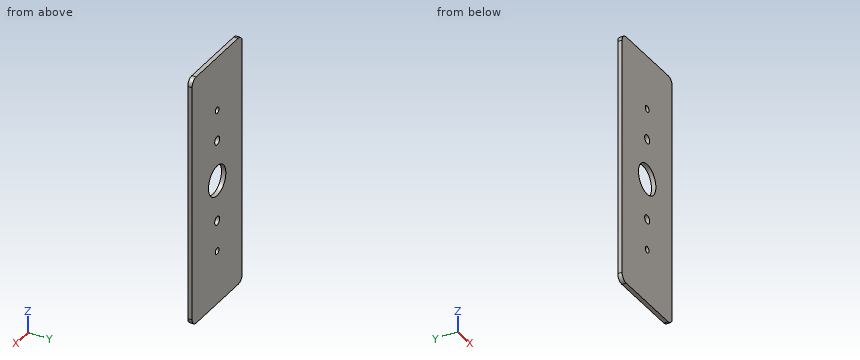
from build123d import *

# Parameters (mm, degrees)
SKETCH1_W               = 30.95625
SKETCH1_H               = 88.9
BOSS_EXTRUDE1_DEPTH     = 1.524
FILLET1_R               = 2.54
SKETCH6_R               = 1.524
CUT_EXTRUDE1_DEPTH      = 2.524
F_4_40_TAPPED_HOLE1_D   = 2.2606
F_1_2_13_TAPPED_HOLE1_D = 10.71626


with BuildPart() as part:
    # Sketch1 → Boss-Extrude1 (new body)
    with BuildSketch(Plane(origin=(0, 0, 0), x_dir=(1, 0, 0), z_dir=(0, 1, 0))):
        Rectangle(SKETCH1_W, SKETCH1_H)
    extrude(amount=BOSS_EXTRUDE1_DEPTH)

    # Fillet1
    fillet1_edges = [part.edges().sort_by_distance(p)[0] for p in [
        (15.478125, 0.762, -44.45),
        (15.478125, 0.762, 44.45),
        (-15.478125, 0.762, 44.45),
        (-15.478125, 0.762, -44.45),
    ]]
    fillet(fillet1_edges, radius=FILLET1_R)

    # Sketch6 → Cut-Extrude1 (cut, through all)
    with BuildSketch(Plane.XZ):
        with Locations((0, 14.478)):
            Circle(SKETCH6_R)
        with Locations((0, -14.478)):
            Circle(SKETCH6_R)
    extrude(amount=-CUT_EXTRUDE1_DEPTH, mode=Mode.SUBTRACT)

    # #4-40 Tapped Hole1 (through all)
    with Locations(Plane(origin=(0, 1.524, 0), x_dir=(-1, 0, 0), z_dir=(0, 1, 0))):
        with Locations((0, 25.4), (0, -25.4)):
            Hole(F_4_40_TAPPED_HOLE1_D / 2)

    # 1/2-13 Tapped Hole1 (through all)
    with Locations(Plane(origin=(0, 1.524, 0), x_dir=(-1, 0, 0), z_dir=(0, 1, 0))):
        with Locations((0, 0)):
            Hole(F_1_2_13_TAPPED_HOLE1_D / 2)


solid = part.part
Can you work these out from the model? Positions are in its coordinate system, mm. Coordinates: 2 decimals unless noted, no trailing zeros. Order: outer loops, then holes, each group sorted by start corner. A loop starts at its lowest first (then second) coordinate and runs counter-clockwise, first axis right, second up. Notation, with made-up numbers: (-25, -14) - (13, -14) arc R3 ccw to (13, -9) - close; hole circle Ø4 at (76, -15.75). An arc over 180 degrees is marked (long way). Answer as a JSON object with one key per item and string values. Group by question number.
Q1. Imagine slicing it at A-A (x = 0). Please give me the cut outline in (y, z), and give its area (3 significant figures).
Q2. Will this pin go through, and if not, where does the flat tip stop? P1, Ø1.8, axis at x = 0, z = 14.478, coming from the -Y side.
Q3. Imagine slicing it at B-B (z = 0). Please give me the cut outline in (x, y), and give its area (3 significant figures).
Q4. Imagine slicing it at C-C (x = -3.5). Please give me the cut outline in (y, z).
Q5. Imagine slicing it at D-D (y = 1.15). Please give me the cut outline in (x, z).
Q6. I need wall thicknesses on line 1 (Z direction, x = 0, y = 0.3); line 2 (Z direction, x = 3, y = 0.85). Which ranges of each line are inside material? Lowest first, please. Write a range as from..to.
Determined:
{
 "1": {"outline": "(0, -44.45) - (1.52, -44.45) - (1.52, -26.53) - (0, -26.53) - close; (0, -24.27) - (1.52, -24.27) - (1.52, -16) - (0, -16) - close; (0, -12.95) - (1.52, -12.95) - (1.52, -5.36) - (0, -5.36) - close; (0, 5.36) - (1.52, 5.36) - (1.52, 12.95) - (0, 12.95) - close; (0, 16) - (1.52, 16) - (1.52, 24.27) - (0, 24.27) - close; (0, 26.53) - (1.52, 26.53) - (1.52, 44.45) - (0, 44.45) - close", "area": "103 mm2"},
 "2": {"P1": "passes through"},
 "3": {"outline": "(-15.48, 0) - (-5.36, 0) - (-5.36, 1.52) - (-15.48, 1.52) - close; (5.36, 0) - (15.48, 0) - (15.48, 1.52) - (5.36, 1.52) - close", "area": "30.8 mm2"},
 "4": {"outline": "(0, -44.45) - (1.52, -44.45) - (1.52, -4.06) - (0, -4.06) - close; (0, 4.06) - (1.52, 4.06) - (1.52, 44.45) - (0, 44.45) - close"},
 "5": {"outline": "(-15.48, -41.91) arc R2.54 ccw to (-12.94, -44.45) - (12.94, -44.45) arc R2.54 ccw to (15.48, -41.91) - (15.48, 41.91) arc R2.54 ccw to (12.94, 44.45) - (-12.94, 44.45) arc R2.54 ccw to (-15.48, 41.91) - close; hole circle Ø10.72 at (0, 0); hole circle Ø3.05 at (0, -14.48); hole circle Ø3.05 at (0, 14.48); hole circle Ø2.26 at (0, -25.4); hole circle Ø2.26 at (0, 25.4)"},
 "6": {"line 1": "z = -44.45..-26.53, -24.27..-16, -12.95..-5.36, 5.36..12.95, 16..24.27, 26.53..44.45", "line 2": "z = -44.45..-4.44, 4.44..44.45"}
}
